Design review of the part built by this model. Coordinates are the model's own, in mm. Coordinates: 2 decimals unless noted, no trailing zeros. Order: outer loops, then holes, each group sorted by start corner. A loop starts at its lowest first (then second) coordinate and runs counter-clockwise, first axis right, second up. Notation, with made-up numbers: (51.25, 22) -> (72.25, 22) arc R19 cw to (72.25, 34) -> close; hole circle Ø5 at (-32, 44.25). An arc over 180 degrees is marked (long way). Use a Markdown table: item, result. Add a question column.
Q1. Wall thickness on probe 1 along Z at (x, y) = (12.7, 4); probe 2 along Z at (x, y) = (38.1, 4.5); probe 3 along X at (y, z) = (7, -14): over which ranges is each line inside the solid? List them lowest first.
Q2. Add section C-C (y = 1.5). Count the separate pieces of the cut face and the enclosed holes in it, then the cut area to 3 significant figures.
Q3. Add section D-D (z = -94.5). State the section outline as (x, y) points (3 decimals), then the cut area to 3 significant figures.
Q4. Insertion check: pin 1 (1.5 mm diameter, centred on x = 34, y = 4.5, fed in from -Z); pin 2 (2 mm diameter, centred on x = 80.5, y = 6.5, fed in from +Z); pin 3 (4 mm diameter, centred on x = 12.7, z = -63.5, fed in from -Y); pin 4 (4 mm diameter, centred on x = 36, y = 1, fed in from -Z). Each pin has a flat end and moves straight along its axis. Give the tip position at first contact, or say it passes through.
Q5. Add section B-B (z = -12.7). State the section outline as (x, y) points (3 decimals), then the cut area to 3 significant figures.
Q6. Add section A-A (x = 88.9). State the section outline as (y, z) points (3 decimals), then the cut area to 3 significant figures.
from build123d import *

# Parameters (mm, degrees)
SKETCH1_W                   = 101.6
SKETCH1_H                   = 127
BOSS_EXTRUDE1_DEPTH         = 9.525
SKETCH2_R                   = 35.052
CUT_EXTRUDE1_DEPTH          = 10.525
F_1_4_CLEARANCE_HOLE1_D     = 6.7564
LPATTERN1_COUNT             = 2
LPATTERN1_PITCH             = 25.4
LPATTERN1_COUNT_DIR2        = 4
LPATTERN1_PITCH_DIR2        = 25.4
TAP_DRILL_FOR_1_4_20_TAP1_D = 5.1054
LPATTERN2_COUNT             = 4
LPATTERN2_PITCH             = 25.4


with BuildPart() as part:
    # Sketch1 → Boss-Extrude1 (new body)
    with BuildSketch(Plane(origin=(0, 0, 0), x_dir=(1, 0, 0), z_dir=(0, 1, 0))):
        with Locations((50.8, 63.5)):
            Rectangle(SKETCH1_W, SKETCH1_H)
    extrude(amount=BOSS_EXTRUDE1_DEPTH)

    # Sketch2 → Cut-Extrude1 (cut, through all)
    with BuildSketch(Plane(origin=(0, 9.525, 0), x_dir=(1, 0, 0), z_dir=(0, 1, 0))):
        with Locations((50.8, 127)):
            Circle(SKETCH2_R)
    extrude(amount=-CUT_EXTRUDE1_DEPTH, mode=Mode.SUBTRACT)

    # 1/4 Clearance Hole1 (through all)
    with Locations(Plane(origin=(0, 9.525, 0), x_dir=(-1, 0, 0), z_dir=(0, 1, 0))):
        with Locations((-12.7, -12.7)):
            f_1_4_clearance_hole1 = Hole(F_1_4_CLEARANCE_HOLE1_D / 2)

    # LPattern1: 1_4 Clearance Hole1 2 × 4
    with Locations(*[(j * LPATTERN1_PITCH_DIR2, 0, -i * LPATTERN1_PITCH) for i in range(LPATTERN1_COUNT) for j in range(LPATTERN1_COUNT_DIR2) if (i, j) != (0, 0)]):
        add(f_1_4_clearance_hole1, mode=Mode.SUBTRACT)

    # Tap Drill for 1/4-20 Tap1 (through all)
    with Locations(Plane(origin=(0, 9.525, 0), x_dir=(-1, 0, 0), z_dir=(0, 1, 0))):
        with Locations((-12.7, -63.5)):
            tap_drill_for_1_4_20_tap1 = Hole(TAP_DRILL_FOR_1_4_20_TAP1_D / 2)

    # LPattern2: Tap Drill for 1/4-20 Tap1 ×4
    with Locations(*[(i * LPATTERN2_PITCH, 0, 0) for i in range(1, LPATTERN2_COUNT)]):
        add(tap_drill_for_1_4_20_tap1, mode=Mode.SUBTRACT)


solid = part.part
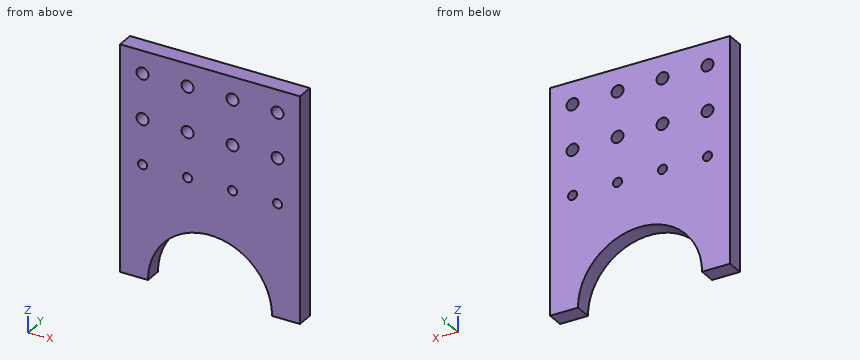
Established:
| question | item | result |
|---|---|---|
| 1 | probe 1 | -127 to -66.05, -60.95 to -41.48, -34.72 to -16.08, -9.32 to 0 |
| 1 | probe 2 | -94.33 to -66.05, -60.95 to -41.48, -34.72 to -16.08, -9.32 to 0 |
| 1 | probe 3 | 0 to 9.58, 15.82 to 34.98, 41.22 to 60.38, 66.62 to 85.78, 92.02 to 101.6 |
| 2 | separate pieces | 1 |
| 2 | enclosed holes | 12 |
| 2 | area | 10,600 mm^2 |
| 3 | outline | (0, 0) -> (37.67, 0) -> (37.67, 9.525) -> (0, 9.525) -> close; (63.93, 0) -> (101.6, 0) -> (101.6, 9.525) -> (63.93, 9.525) -> close |
| 3 | area | 718 mm^2 |
| 4 | pin 1 | z = -96.66 |
| 4 | pin 2 | z = 0 |
| 4 | pin 3 | through |
| 4 | pin 4 | z = -96.24 |
| 5 | outline | (0, 0) -> (9.322, 0) -> (9.322, 9.525) -> (0, 9.525) -> close; (16.078, 0) -> (34.722, 0) -> (34.722, 9.525) -> (16.078, 9.525) -> close; (41.478, 0) -> (60.122, 0) -> (60.122, 9.525) -> (41.478, 9.525) -> close; (66.878, 0) -> (85.522, 0) -> (85.522, 9.525) -> (66.878, 9.525) -> close; (92.278, 0) -> (101.6, 0) -> (101.6, 9.525) -> (92.278, 9.525) -> close |
| 5 | area | 710 mm^2 |
| 6 | outline | (0, -127) -> (9.525, -127) -> (9.525, -66.053) -> (0, -66.053) -> close; (0, -60.947) -> (9.525, -60.947) -> (9.525, -41.478) -> (0, -41.478) -> close; (0, -34.722) -> (9.525, -34.722) -> (9.525, -16.078) -> (0, -16.078) -> close; (0, -9.322) -> (9.525, -9.322) -> (9.525, 0) -> (0, 0) -> close |
| 6 | area | 1,030 mm^2 |
